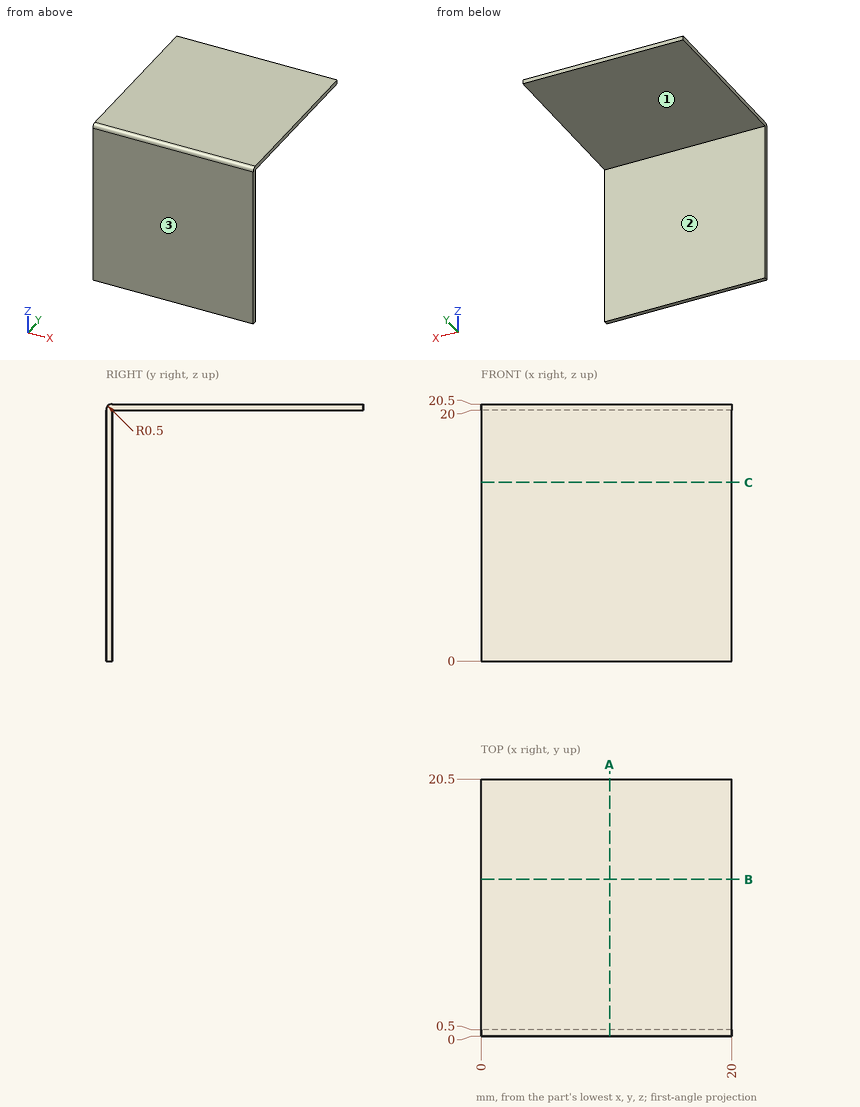
Here's the drawing with two shaded views (mm, measured from the low corner). I have some questions. Coordinates: 2 decimals unless noted, no trailing zeros. Write each loop counter-clockwise with the first axis right and the second up, starting at its lowest first coordinate (ties: lowest second). Pieces come first, ordered by that corner, then holes.
Item 1: Will these pins go through, and if not, where does the flat tip stop? pin 1 (6 mm diameter, centred on x = 5, z = 13, fed in from +Y); pin 2 (1.5 mm diameter, centred on x = 15, y = 6.5, fed in from -Z).
Item 2: I want a section at A-A on x = 10.25. Write out the boundary of the cut face in (y, z), and give its area (3 significant figures).
Item 3: If I drill on line 1 (Y direction, x = 10, z = 2.25); line 2 (Z direction, x = 13.75, y = 15.5), over which ranges is the centre line in solid material (lowest first)?
Item 4: If we mould it in two halves opening along Y, with no side actions, what happens to the marked faces 1, 2 and 3? For each: +Y half, -Y half, draft (parallel to the pull), parting line (faces both ways), or undercut.
Item 5: I want a section at B-B on y = 12.5. Write out the boundary of the cut face in (x, z), and give its area (3 significant figures).
Item 6: I want a section at C-C on z = 14.25. Write out the boundary of the cut face in (x, y).
Findings below:
1. pin 1: stops at y = 0.5
1. pin 2: stops at z = 20
2. outline: (0, 0) - (0.5, 0) - (0.5, 20) - (20.5, 20) - (20.5, 20.5) - (0.5, 20.5) arc R0.5 ccw to (0, 20) - close
2. area: 20.2 mm2
3. line 1: y = 0 to 0.5
3. line 2: z = 20 to 20.5
4. face 1: draft
4. face 2: +Y half
4. face 3: -Y half
5. outline: (0, 20) - (20, 20) - (20, 20.5) - (0, 20.5) - close
5. area: 10.0 mm2
6. outline: (0, 0) - (20, 0) - (20, 0.5) - (0, 0.5) - close
